Verification items for the finished model (mm, model axes). Face numbers are marked on the shaded views. Coordinates: 2 decimals unless noted, no trailing zeros. Order: outer loops, then holes, each group sorted by start corner. A loop starts at its lowest first (then second) coordinate and runs counter-clockwise, first axis right, second up. Notation, with made-up numbers: (67, -27) -> (87, -27) arc R9 ccw to (87, -17) -> close; hole circle Ø3 at (70.5, 62). An arc over 180 degrees is marked (long way). Use CSV: the item, a comma, the result in double quotes. Start each with the question number.
1) Sectioned sample at C-C on x = -83.5. Record the boundary of the cut face in (y, z), then the cut area to 3 significant figures.
2) Sectioned sample at D-D on z = 3.75. Give the number of separate pieces and of enclosed holes in the cut face, then the cut area to 3 significant figures.
3) Go/stop test with flat-tipped pins: pin 1 (4.5 mm diameter, centred on x = -158.115, y = 45.72, fed in from +Z); pin 2 (5 mm diameter, centred on x = -60, y = 14.5, fed in from +Z); pin 3 (6.5 mm diameter, centred on x = -16.51, y = 4.55, fed in from -Z). Record where each tip stops, or that it passes through.
4) Scan lines: line 1 along Y through (x, z) = (-118, 5.75); line 2 along Y through (x, z) = (-68, 4.5); line 3 along Z through (x, y) = (-152.5, 19). Record each from-to range of solid material in increasing order.
5) Sectioned sample at A-A on y = 45.72. Record the boundary of the cut face in (x, z).
6) Sectioned sample at B-B on x = -16.51. Record the boundary of the cut face in (y, z).
7) Release check for a two-part mould opening along Y. For the marked faces 1 and 2 record: released by +Y, released by -Y, zero draft, split by the parting line, or undercut.
from build123d import *

# Parameters (mm, degrees)
SKETCH5_W                    = 235.204
SKETCH5_H                    = 50.8
BOSS_EXTRUDE3_DEPTH          = 7.62
CUT_EXTRUDE3_DEPTH           = 6.35
F_10_0_1935_DIAMETER_HOLE1_D = 4.9149


with BuildPart() as part:
    # Sketch5 → Boss-Extrude3 (new body)
    with BuildSketch(Plane.XY):
        with Locations((-117.602, 25.4)):
            Rectangle(SKETCH5_W, SKETCH5_H)
    extrude(amount=BOSS_EXTRUDE3_DEPTH)

    # Sketch6 → Cut-Extrude3 (cut)
    with BuildSketch(Plane.XY.offset(7.62)):
        with BuildLine():
            Line((-57.912, 9.652), (-186.436, 9.652))
            ThreePointArc((-186.436, 9.652), (-200.66, 23.876), (-186.436, 38.1))
            Line((-186.436, 38.1), (-57.912, 38.1))
            ThreePointArc((-57.912, 38.1), (-43.688, 23.876), (-57.912, 9.652))
        make_face()
    extrude(amount=-CUT_EXTRUDE3_DEPTH, mode=Mode.SUBTRACT)

    # #10 (0.1935) Diameter Hole1 (through all)
    with Locations(Plane(origin=(-198.501, 45.72, 7.62), x_dir=(1, 0, 0), z_dir=(0, 0, 1))):
        with Locations((0, 0), (40.386, 0), (80.772, 0), (121.158, 0), (161.544, 0), (-20.193, -41.171520692), (20.2438, -41.171520692), (60.6806, -41.171520692), (101.1174, -41.171520692), (141.5542, -41.171520692), (181.991, -41.171520692)):
            Hole(F_10_0_1935_DIAMETER_HOLE1_D / 2)


solid = part.part
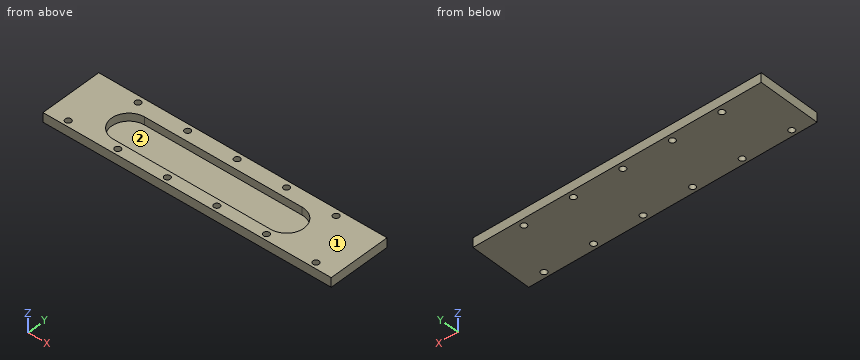
Answers follow:
1,outline,"(0, 0) -> (50.8, 0) -> (50.8, 7.62) -> (38.1, 7.62) -> (38.1, 1.27) -> (9.65, 1.27) -> (9.65, 7.62) -> (0, 7.62) -> close"
1,area,"206 mm²"
2,separate pieces,"1"
2,enclosed holes,"12"
2,area,"7,450 mm²"
3,pin 1,"passes through"
3,pin 2,"stops at z = 1.27"
3,pin 3,"stops at z = 0"
4,line 1,"y = 0 to 9.65, 38.1 to 43.28, 48.16 to 50.8"
4,line 2,"y = 0 to 9.65, 38.1 to 50.8"
4,line 3,"z = 0 to 1.27"
5,outline,"(-235.2, 0) -> (-200.96, 0) -> (-200.96, 7.62) -> (-235.2, 7.62) -> close; (-196.04, 0) -> (-160.57, 0) -> (-160.57, 7.62) -> (-196.04, 7.62) -> close; (-155.66, 0) -> (-120.19, 0) -> (-120.19, 7.62) -> (-155.66, 7.62) -> close; (-115.27, 0) -> (-79.8, 0) -> (-79.8, 7.62) -> (-115.27, 7.62) -> close; (-74.89, 0) -> (-39.41, 0) -> (-39.41, 7.62) -> (-74.89, 7.62) -> close; (-34.5, 0) -> (0, 0) -> (0, 7.62) -> (-34.5, 7.62) -> close"
6,outline,"(0, 0) -> (2.09, 0) -> (2.09, 7.62) -> (0, 7.62) -> close; (7.01, 0) -> (50.8, 0) -> (50.8, 7.62) -> (7.01, 7.62) -> close"
7,face 1,"zero draft"
7,face 2,"undercut"
